Autodesk Inventor part; units mm, degrees
ref_plane "YZ Plane" through (0, 0, 0) normal (1, 0, 0) x (0, 1, 0)
ref_plane "XZ Plane" through (0, 0, 0) normal (0, 1, 0) x (-1, 0, 0)
ref_plane "XY Plane" through (0, 0, 0) normal (0, 0, 1) x (1, 0, 0)
sketch "Sketch1" plane through (0, 0, 0) normal (1, 0, 0) x (0, 1, 0)
  circle A0 centre (0, 0) radius 5.7227
extrude "Extrusion1" add sketch "Sketch1" along normal blind 1
sketch "Sketch2" plane through (1, 0, 0) normal (1, 0, 0) x (0, 0, -1)
  circle A0 centre (0, 0) radius 6.7072
extrude "Extrusion2" add sketch "Sketch2" along normal blind 0.5
sketch "Sketch3" plane through (0, 0, 0) normal (-1, 0, 0) x (0, 0, 1)
  circle A0 centre (-0.1652, 0) radius 0.512
  point P0 (0, 0)
extrude "Extrusion3" add sketch "Sketch3" along normal blind 3
The listing builds one solid part. Answer for the finished solid, in the listing's coordinates (mm). A direction names the side the tool comes from. Give positions to 0.01 mm unless a question says otherwise; leave off trailing zeros. Order: outer loops, then holes, each group sorted by start corner. A loop starts at its lowest first (then second) coordinate and runs counter-clockwise, first axis right, second up. Notation, with made-up numbers: (62, 74) -> (117, 74) arc R13 ccw to (117, 80) -> close; hole circle Ø8 at (63, 6.5). An arc over 180 degrees is marked (long way). Answer as a JSON object with one key per item and string values. Group by question number.
Item 1: Determine the mould class of faces 1 (the flat face through (1.5, 0, 0)), 2 (the cylindrical face through (1.25, 6.55, 1.45)), 3 (the flat face through (0, 0, -1)) for opening direction X: pulls with the +X half, pulls with the -X half, needs draft (parallel to the pull), parting line crosses it, or undercut.
Item 2: The part is cut by section B-B on z = -1.25. Write down the section's boundary in (x, y), and give its area (3 significant figures).
Item 3: Consider L1, parallel to X at y = -0.25, z = -4; L2, parallel to X at y = 2.5, z = 5.75; L3, parallel to Y at x = 0.8, z = -0.75. Determine where each line is inside the solid, lowest interval first. Write a range as from..to.
Item 4: Flat-ended cylindrical pins translate along their axes: pin 1 (5 mm diameter, centred on y = 1.5, z = -3, fed in from -X); pin 2 (2 mm diameter, centred on x = 1, z = -2, fed in from -Y); pin 3 (2 mm diameter, centred on x = 1, z = -4, fed in from -Y). Find the tip coordinate at first contact, or state that the pin passes through.
Item 5: The part is cut by section D-D on y = 2.5. Write down the section's boundary in (x, z).
Item 6: A tool of negligible diameter and unlimited length cuts with its end or side. For faces 4 (the flat face through (-3, 0, 0)), 5 (the cylindrical face through (0.493, -1.241, 5.587)), from which of +Z, -Z, +X, -X, +Y, -Y can it reach the whole face along a straight path? Write none if from no direction.
Item 7: The part is cut by section A-A on y = 0. Write down the section's boundary in (x, z).
Item 8: The part is cut by section C-C on x = -0.9. Write down the section's boundary in (y, z), and give its area (3 significant figures).
Result set:
{
 "1": {"face 1": "pulls with the +X half", "face 2": "needs draft", "face 3": "pulls with the -X half"},
 "2": {"outline": "(0, -5.58) -> (1, -5.58) -> (1, -6.59) -> (1.5, -6.59) -> (1.5, 6.59) -> (1, 6.59) -> (1, 5.58) -> (0, 5.58) -> close", "area": "17.8 mm²"},
 "3": {"L1": "0..1.5", "L2": "1..1.5", "L3": "-5.67..5.67"},
 "4": {"pin 1": "x = 0", "pin 2": "y = -6.63", "pin 3": "y = -6"},
 "5": {"outline": "(0, -5.15) -> (1, -5.15) -> (1, -6.22) -> (1.5, -6.22) -> (1.5, 6.22) -> (1, 6.22) -> (1, 5.15) -> (0, 5.15) -> close"},
 "6": {"face 4": "+Z, -Z, -X, +Y, -Y", "face 5": "-X"},
 "7": {"outline": "(-3, -0.68) -> (0, -0.68) -> (0, -5.72) -> (1, -5.72) -> (1, -6.71) -> (1.5, -6.71) -> (1.5, 6.71) -> (1, 6.71) -> (1, 5.72) -> (0, 5.72) -> (0, 0.35) -> (-3, 0.35) -> close"},
 "8": {"outline": "circle Ø1.02 at (0, -0.17)", "area": "0.824 mm²"}
}
